```python
from build123d import *

# Parameters (mm, degrees)
SKETCH1_W                                        = 40
SKETCH1_H                                        = 10
BOSS_EXTRUDE1_DEPTH                              = 3
CBORE_FOR_M3_PAN_HEAD_MACHINE_SCREW1_D           = 3.4
CBORE_FOR_M3_PAN_HEAD_MACHINE_SCREW1_DEPTH       = 3
CBORE_FOR_M3_PAN_HEAD_MACHINE_SCREW1_CBORE_D     = 7.5
CBORE_FOR_M3_PAN_HEAD_MACHINE_SCREW1_CBORE_DEPTH = 0.5


with BuildPart() as part:
    # Sketch1 → Boss-Extrude1 (new body)
    with BuildSketch(Plane(origin=(0, 0, 0), x_dir=(1, 0, 0), z_dir=(0, 1, 0))):
        with Locations((20, -5)):
            Rectangle(SKETCH1_W, SKETCH1_H)
    extrude(amount=-BOSS_EXTRUDE1_DEPTH)

    # CBORE for M3 Pan Head Machine Screw1
    with Locations(Plane(origin=(0, 0, 0), x_dir=(1, 0, 0), z_dir=(0, 1, 0))):
        with Locations((4, -5), (36, -5)):
            CounterBoreHole(CBORE_FOR_M3_PAN_HEAD_MACHINE_SCREW1_D / 2, CBORE_FOR_M3_PAN_HEAD_MACHINE_SCREW1_CBORE_D / 2, CBORE_FOR_M3_PAN_HEAD_MACHINE_SCREW1_CBORE_DEPTH, depth=CBORE_FOR_M3_PAN_HEAD_MACHINE_SCREW1_DEPTH)


solid = part.part
```
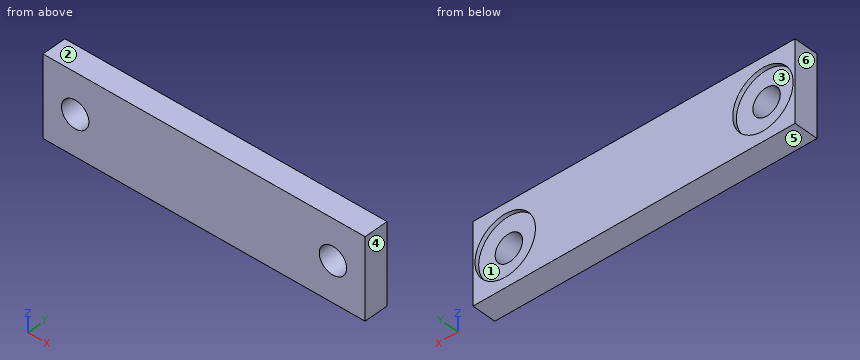
CAD build for the part. Positions are in the model's coordinates, mm. Face numbers are marked on the shaded views. A direction names the side the tool comes from. Coordinates: 2 decimals unless noted, no trailing zeros. Loops run counter-clockwise (first coordinate to the right, second up) from the corner with the lowest first, then second, coordinate; pieces in that order, holes last. Notation, with made-up numbers: (41, -5) - (45, -5) arc R27 ccw to (45, 34) - close; hole circle Ø5 at (0.5, -34.5). An arc over 180 degrees is marked (long way). Use CSV: the item, a comma, the result in double quotes. Start each with the question number.
Q1. Cut at C-C, the plane z = 5. List the corners of the cut face in (x, y), then the cut area to 3 significant figures.
Q2. Cut at B-B, the plane y = -1.8. List the corners of the cut face in (x, z), then the cut area to 3 significant figures.
Q3. Cut at A-A, the plane x = 36. List the corners of the cut face in (y, z).
Q4. Probe probe 1 along X at (y, z) = (-1.4, 5); probe 2 along Z at (x, y) = (36, -1.65); probe 3 along X at (y, z) = (-0.15, 8). List the from-to ranges inside material, lowest first. Write a range as from..to.
Q5. Two-plate mould, pull along X, no slides. Class the marked faces 3, 4, 5 and 6: +X half, -X half, draft (parallel to the pull), parting line (faces both ways), or undercut.
Q6. 3-axis set-ups, long thin cutter, end or side, ignore diameter. For the marked faces 1 and 2: which of +Z, -Z, +X, -X, +Y, -Y reach the whole face in a straight line?
Q7. Cut at D-D, the plane z = 2.5. List the corners of the cut face in (x, y), then the cut area to 3 significant figures.
Q8. Drop a flat-ended pin along its axis: P1, Ø4.5, axis at x = 4, z = 5, coming from the +Y side. Give the stop position or say it passes through.
Here are the results:
1,outline,"(0, -3) - (2.3, -3) - (2.3, -0.5) - (0.25, -0.5) - (0.25, 0) - (0, 0) - close; (5.7, -3) - (34.3, -3) - (34.3, -0.5) - (32.25, -0.5) - (32.25, 0) - (7.75, 0) - (7.75, -0.5) - (5.7, -0.5) - close; (37.7, -3) - (40, -3) - (40, 0) - (39.75, 0) - (39.75, -0.5) - (37.7, -0.5) - close"
1,area,"95.5 mm2"
2,outline,"(0, 0) - (40, 0) - (40, 10) - (0, 10) - close; hole circle Ø3.4 at (4, 5); hole circle Ø3.4 at (36, 5)"
2,area,"382 mm2"
3,outline,"(-3, 0) - (0, 0) - (0, 1.25) - (-0.5, 1.25) - (-0.5, 3.3) - (-3, 3.3) - close; (-3, 6.7) - (-0.5, 6.7) - (-0.5, 8.75) - (0, 8.75) - (0, 10) - (-3, 10) - close"
4,probe 1,"0..2.3, 5.7..34.3, 37.7..40"
4,probe 2,"0..3.3, 6.7..10"
4,probe 3,"0..1.75, 6.25..33.75, 38.25..40"
5,face 3,"undercut"
5,face 4,"+X half"
5,face 5,"draft"
5,face 6,"-X half"
6,face 1,"+Y"
6,face 2,"+Z, +X, -X, +Y, -Y"
7,outline,"(0, -3) - (40, -3) - (40, 0) - (38.8, 0) - (38.8, -0.5) - (33.2, -0.5) - (33.2, 0) - (6.8, 0) - (6.8, -0.5) - (1.2, -0.5) - (1.2, 0) - (0, 0) - close"
7,area,"114 mm2"
8,P1,"y = -0.5"
